For this review, take the finished solid that the model builds, in its own axes (mm). A direction names the side the tool comes from. Coordinates: 2 decimals unless noted, no trailing zeros. Order: outer loops, then holes, each group sorted by start corner. A loop starts at its lowest first (then second) coordinate and runs counter-clockwise, first axis right, second up. Notation, with made-up numbers: (52, 55.25) - (61, 55.25) arc R19 cw to (61, 62.25) - close; hole circle Ø3 at (-33.5, 35.25). An arc over 180 degrees is marked (long way). One line per item, written item: value. Start each with the question number.
(1) For faces 1 (the flat face through (-1, -493, 120)), 2 (the flat face through (-1, -493, 125)), 3 (the cylindrical face through (13.38, -275.73, 122.54)), list the 3-axis set-ups (+Z, -Z, +X, -X, +Y, -Y) from which the entire face can be reached by the end or side of a thin tool; tool diameter is ignored.
(2) Mouldability with a two-part tool opening along Z and no side actions: class faces 4 (the flat face through (-1, -493, -125)), 5 (the flat face through (48, 0, 38)), 6 (the flat face through (45, -493, -2)) as released by +Z, released by -Z, zero draft, split by the parting line, or undercut.
(3) Consider section A-A on y = -950. Write out the cut boundary in (x, z).
(4) Consider section B-B on z = -13.5. Write out the cut boundary in (x, y), then the cut area to 3 significant figures.
(5) To check wall thickness, follow line 1 along Y through (x, z) = (0, 123); line 2 along Z through (x, y) = (-40.5, -396); line 3 along X through (y, z) = (-247, 91). State the ranges of each line that lie inside material, in increasing order.
(6) Consider section D-D on z = -75. Write out the cut boundary in (x, y).
(7) Consider section C-C on x = 0. Write out the cut boundary in (y, z).
```python
from build123d import *

# Parameters (mm, degrees)
F0_W     = 100
F0_H     = 250
F0_W_2   = 90
F0_H_2   = 240
F1_DEPTH = 1000
F2_R     = 10
F3_DEPTH = 100.001
F4_R     = 29
F5_R     = 29
F6_DEPTH = 5
F7_W     = 26
F7_H     = 26
F8_DEPTH = 250.001


# Not quite as in the source:
# - a feature names something its author has since deleted; it is built from what else it names


with BuildPart() as f1:
    # F0 (on Front) → F1 (new body)
    with BuildSketch(Plane.XZ):
        Rectangle(F0_W, F0_H)
        Rectangle(F0_W_2, F0_H_2, mode=Mode.SUBTRACT)
    extrude(amount=F1_DEPTH)

    # F2 (on face) → F3 (cut, through all)
    with BuildSketch(Plane.YZ.offset(50)):
        with Locations((-950, -75)):
            Circle(F2_R)
    extrude(amount=-F3_DEPTH, mode=Mode.SUBTRACT)

    # F4 (on face) + F5 (on face) → F6 (cut, through all)
    with BuildSketch(Plane.XY.offset(125)):
        with Locations((0, -800)):
            Circle(F4_R)
    with BuildSketch(Plane.XY.offset(125)):
        with Locations((0, -250)):
            Circle(F5_R)
    extrude(amount=-F6_DEPTH, mode=Mode.SUBTRACT)

    # F7 (on face) → F8 (cut, through all)
    with BuildSketch(Plane.XY.offset(125)):
        with Locations((0, -900)):
            Rectangle(F7_W, F7_H)
    extrude(amount=-F8_DEPTH, mode=Mode.SUBTRACT)


solid = f1.part
```
Geometry check:
1. face 1: +Y, -Y
1. face 2: +Z, +X, -X, +Y, -Y
1. face 3: +Z
2. face 4: released by -Z
2. face 5: zero draft
2. face 6: undercut
3. outline: (-50, -125) - (50, -125) - (50, -85) - (45, -85) - (45, -120) - (-45, -120) - (-45, -85) - (-50, -85) - close; (-50, -65) - (-45, -65) - (-45, 120) - (45, 120) - (45, -65) - (50, -65) - (50, 125) - (-50, 125) - close
4. outline: (-50, -1000) - (-45, -1000) - (-45, 0) - (-50, 0) - close; (45, -1000) - (50, -1000) - (50, 0) - (45, 0) - close
4. area: 10,000 mm^2
5. line 1: y = -1000 to -913, -887 to -829, -771 to -279, -221 to 0
5. line 2: z = -125 to -120, 120 to 125
5. line 3: x = -50 to -45, 45 to 50
6. outline: (-50, -1000) - (-45, -1000) - (-45, -960) - (-50, -960) - close; (-50, -940) - (-45, -940) - (-45, 0) - (-50, 0) - close; (45, -1000) - (50, -1000) - (50, -960) - (45, -960) - close; (45, -940) - (50, -940) - (50, 0) - (45, 0) - close
7. outline: (-1000, -125) - (-913, -125) - (-913, -120) - (-1000, -120) - close; (-1000, 120) - (-913, 120) - (-913, 125) - (-1000, 125) - close; (-887, -125) - (0, -125) - (0, -120) - (-887, -120) - close; (-887, 120) - (-829, 120) - (-829, 125) - (-887, 125) - close; (-771, 120) - (-279, 120) - (-279, 125) - (-771, 125) - close; (-221, 120) - (0, 120) - (0, 125) - (-221, 125) - close
